Could you check a few things on this model? Use its own coordinates, in mm. A direction names the side the tool comes from. Round coordinates to 2 decimals unless told otherwise and drop trailing zeros. Answer in a Markdown table with one row per item.
from build123d import *

# Parameters (mm, degrees)
F0_R     = 2.032
F0_R_2   = 1.2446
F1_DEPTH = 3.175
F2_R     = 3.175
F3_DEPTH = 3.175
F4_R     = 4.7625
F5_DEPTH = 25.4
F6_R     = 3.96875
F7_DEPTH = 76.2
F9_D     = 6.35
F9_DEPTH = 100.33
F9_TIP   = 1.9077324654
F10_D    = 2.4892
F11_SIZE = 0.508


with BuildPart() as f1:
    # F0 (on Front) → F1 (new body)
    with BuildSketch(Plane.XZ):
        Circle(F0_R)
        Circle(F0_R_2, mode=Mode.SUBTRACT)
    extrude(amount=F1_DEPTH)

    # F2 (on face) → F3 (join)
    with BuildSketch(Plane.XZ.offset(3.175)):
        Circle(F2_R)
    extrude(amount=F3_DEPTH)

    # F4 (on face) → F5 (join)
    with BuildSketch(Plane.XZ.offset(6.35)):
        Circle(F4_R)
    extrude(amount=F5_DEPTH)

    # F6 (on face) → F7 (join)
    with BuildSketch(Plane.XZ.offset(31.75)):
        Circle(F6_R)
    extrude(amount=F7_DEPTH)

    # F9
    with Locations(Plane.XZ.offset(107.95)):
        with Locations((0, 0)):
            Hole(F9_D / 2, depth=F9_DEPTH)
            with Locations((0, 0, -(F9_DEPTH + F9_TIP / 2))):  # 118° drill point
                Cone(0, F9_D / 2, F9_TIP, mode=Mode.SUBTRACT)

    # F10 (through all)
    with Locations(Plane.XZ.offset(107.95)):
        with Locations((0, 0)):
            Hole(F10_D / 2)

    # F11
    f11_edges = [f1.edges().sort_by_distance(p)[0] for p in [
        (-2.032, 0, 0),
        (-3.175, -3.175, 0),
        (-4.7625, -6.35, 0),
        (-4.7625, -31.75, 0),
        (-3.96875, -107.95, 0),
    ]]
    chamfer(f11_edges, length=F11_SIZE)


solid = f1.part
1) For faces 4 (the face through (-0.86, -69.066, -3.874)), 5 (the face through (-1, -3.175, -2)), 6 (the face through (-3.78, -18.88, -2.9)), which set-ups out of +Z, -Z, +X, -X, +Y, -Y let a thin tool reach every point of the face, with its end or its side?
Findings:
| item | result |
|---|---|
| face 4 | -Y |
| face 5 | +Y |
| face 6 | +Y, -Y |
2) Please list where these lines run through material, in increasing order: line 1 (Z direction, x = 0, y = -64) (3 decimals); line 2 (Z direction, x = 0, y = -3.95) (3 decimals); line 3 (X direction, y = -57, z = 0.75).
Findings:
| item | result |
|---|---|
| line 1 | z = -3.969 to -3.175, 3.175 to 3.969 |
| line 2 | z = -3.175 to -1.245, 1.245 to 3.175 |
| line 3 | x = -3.9 to -3.09, 3.09 to 3.9 |
3) For pin 1 (1 mm diameter, centred on x = 4, z = -2.5, fed in from -Y); pin 2 (3 mm diameter, centred on x = -2.5, z = 2.5, fed in from -Y); pin 3 (2 mm diameter, centred on y = -65.5, z = -1.5, fed in from -X); pin 4 (2 mm diameter, centred on x = 1.5, z = 1, fed in from -Y), each with a flat end and sliding along its axis, tell me the tip position at first contact or that it passes through.
Findings:
| item | result |
|---|---|
| pin 1 | stops at y = -31.75 |
| pin 2 | stops at y = -107.95 |
| pin 3 | stops at x = -3.94 |
| pin 4 | stops at y = -7.4 |
4) Thinking about a two-plate mould opening in Z: for faces 1 (the face through (-0.69, -5, -3.1)), 2 (the face through (-2, -6.35, -3)), 3 (the face through (0.69, -57.08, -3.1)), which applies, +Z half, -Z half, draft (parallel to the pull), parting line (faces both ways), or undercut?
Findings:
| item | result |
|---|---|
| face 1 | parting line |
| face 2 | draft |
| face 3 | undercut |
